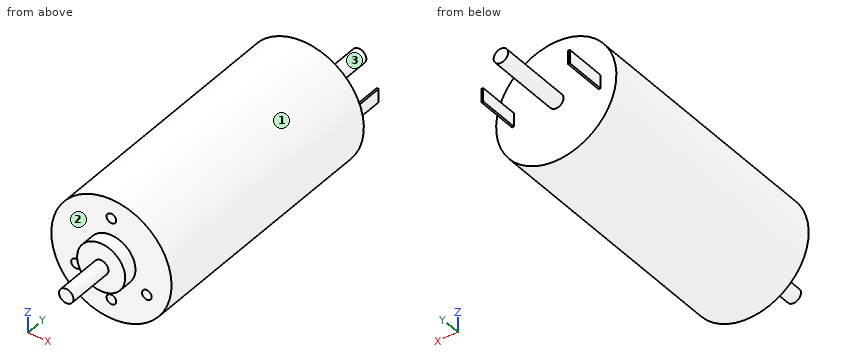
```python
from build123d import *

# Parameters (mm, degrees)
SKETCH1_R           = 12.5
BOSS_EXTRUDE1_DEPTH = 54.5
SKETCH2_R           = 1.5
BOSS_EXTRUDE2_DEPTH = 12.8
BOSS_EXTRUDE3_START = 15.7
SKETCH3_R           = 1.5
BOSS_EXTRUDE3_DEPTH = 15.7
SKETCH4_W           = 0.4
SKETCH4_H           = 2.8
BOSS_EXTRUDE4_DEPTH = 8.7
SKETCH5_R           = 1
CUT_EXTRUDE1_DEPTH  = 2.9
SKETCH6_R           = 5
BOSS_EXTRUDE5_DEPTH = 2.9


with BuildPart() as part:
    # Sketch1 → Boss-Extrude1 (new body)
    with BuildSketch(Plane(origin=(0, 0, 0), x_dir=(1, 0, 0), z_dir=(0, 1, 0))):
        with Locations(Location((0, 0, 0), (0, 0, 270))):
            Circle(SKETCH1_R)
    extrude(amount=-BOSS_EXTRUDE1_DEPTH)

    # Sketch2 → Boss-Extrude2 (add)
    with BuildSketch(Plane.XZ.offset(54.5)):
        with Locations(Location((0, 0, 0), (0, 0, 90))):
            Circle(SKETCH2_R)
    extrude(amount=BOSS_EXTRUDE2_DEPTH)

    # Sketch3 → Boss-Extrude3 (add)
    with BuildSketch(Plane(origin=(0, 0, 0), x_dir=(1, 0, 0), z_dir=(0, 1, 0)).offset(BOSS_EXTRUDE3_START)):
        with Locations(Location((0, 0, 0), (0, 0, 270))):
            Circle(SKETCH3_R)
    extrude(amount=-BOSS_EXTRUDE3_DEPTH)

    # Sketch4 → Boss-Extrude4 (add)
    with BuildSketch(Plane(origin=(0, 0, 0), x_dir=(1, 0, 0), z_dir=(0, 1, 0))):
        with Locations((9, 0)):
            Rectangle(SKETCH4_W, SKETCH4_H)
        with Locations((-9, 0)):
            Rectangle(SKETCH4_W, SKETCH4_H)
    extrude(amount=BOSS_EXTRUDE4_DEPTH)

    # Sketch5 → Cut-Extrude1 (cut)
    with BuildSketch(Plane.XZ.offset(54.5)):
        with Locations(Location((0, 8.5, 0), (0, 0, 270))):
            Circle(SKETCH5_R)
        with Locations(Location((0, -8.5, 0), (0, 0, 270))):
            Circle(SKETCH5_R)
        with Locations(Location((-7.361215932, -4.25, 0), (0, 0, 270))):
            Circle(SKETCH5_R)
        with Locations(Location((7.361215932, -4.25, 0), (0, 0, 90))):
            Circle(SKETCH5_R)
    extrude(amount=-CUT_EXTRUDE1_DEPTH, mode=Mode.SUBTRACT)

    # Sketch6 → Boss-Extrude5 (add)
    with BuildSketch(Plane.XZ.offset(54.5)):
        with Locations(Location((0, 0, 0), (0, 0, 90))):
            Circle(SKETCH6_R)
    extrude(amount=BOSS_EXTRUDE5_DEPTH)


solid = part.part
```
The model under review builds one solid part; all positions refer to its coordinate system, in mm. Face numbers are marked on the shaded views. A direction names the side the tool comes from. Coordinates: 2 decimals unless noted, no trailing zeros. Loops run counter-clockwise (first coordinate to the right, second up) from the corner with the lowest first, then second, coordinate; pieces in that order, holes last. Notation, with made-up numbers: (21, 33) -> (31, 33) arc R17 ccw to (31, 63) -> close; hole circle Ø7 at (43, -36.5). An arc over 180 degrees is marked (long way). Answer as CSV lines item,"result".
Item 1: Take a section at A-A, the plane y = 6.5. State the section outline as (x, z) points.
Results below:
outline,"(-9.2, -1.4) -> (-8.8, -1.4) -> (-8.8, 1.4) -> (-9.2, 1.4) -> close; circle Ø3 at (0, 0); (8.8, -1.4) -> (9.2, -1.4) -> (9.2, 1.4) -> (8.8, 1.4) -> close"
Item 2: Machinability: for the marked faces 1, 2 and 3, which of the approach directions +Z, -Z, +X, -X, +Y, -Y give a long, thin tool a straight path to every point of the face, cutting with its end or side? Answer none if there is none.
Results below:
face 1,"+Y, -Y"
face 2,"-Y"
face 3,"+Y"
Item 3: Insertion check: pin 1 (1.2 mm diameter, centred on x = 0, z = -8.5, fed in from -Y); pin 2 (5 mm diameter, centred on x = -1, z = -8.5, fed in from +Y); pin 3 (1 mm diameter, centred on x = 8, z = -9.5, fed in from -Y). Each pin has a flat end and moves straight along its axis. Give the tip position at first contact, or say it passes through.
Results below:
pin 1,"stops at y = -51.6"
pin 2,"stops at y = 0"
pin 3,"stops at y = -54.5"
Item 4: Take a section at C-C, the plane y = -31. State the section outline as (x, z) points, and give its area (3 significant figures).
Results below:
outline,"circle Ø25 at (0, 0)"
area,"491 mm2"
Item 5: Take a section at B-B, the plane z = 0. State the section outline as (x, y) points, and give its area (3 significant figures).
Results below:
outline,"(-12.5, -54.5) -> (-5, -54.5) -> (-5, -57.4) -> (-1.5, -57.4) -> (-1.5, -67.3) -> (1.5, -67.3) -> (1.5, -57.4) -> (5, -57.4) -> (5, -54.5) -> (12.5, -54.5) -> (12.5, 0) -> (9.2, 0) -> (9.2, 8.7) -> (8.8, 8.7) -> (8.8, 0) -> (1.5, 0) -> (1.5, 15.7) -> (-1.5, 15.7) -> (-1.5, 0) -> (-8.8, 0) -> (-8.8, 8.7) -> (-9.2, 8.7) -> (-9.2, 0) -> (-12.5, 0) -> close"
area,"1,480 mm2"
Item 6: Take a section at D-D, the plane x = 3.75. State the section outline as (y, z) points, and give its area (3 significant figures).
Results below:
outline,"(-57.4, -3.31) -> (-54.5, -3.31) -> (-54.5, -11.92) -> (0, -11.92) -> (0, 11.92) -> (-54.5, 11.92) -> (-54.5, 3.31) -> (-57.4, 3.31) -> close"
area,"1,320 mm2"
Item 7: For L1, parallel to Z at x = -0.5, y = -2; L2, parallel to Y at x = 9.25, z = -4; L3, parallel to Z at x = -8.25, y = -52.5, list the stretches that pass through material, from the lowest coordinate up.
Results below:
L1,"z = -12.49 to 12.49"
L2,"y = -54.5 to 0"
L3,"z = -9.39 to -4.71, -3.79 to 9.39"
